Input: part model. Units: mm. Frame: model coordinates. A direction names the side the tool comes from. Give positions to 0.01 mm unless a question says otherwise; leave off trailing zeros. Loops run counter-clockwise (first coordinate to the right, second up) from the corner with the lowest first, then second, coordinate; pieces in that order, holes last. Notation, with made-up numbers: (60, 10.25) - (116, 10.25) arc R21 ccw to (116, 39.25) - close; hole circle Ø10 at (71, 58.25). An arc over 180 degrees is marked (long way). One line per item, written item: value.
from build123d import *

# Parameters (mm, degrees)
SKETCH1_R              = 6.35
SKETCH1_R_2            = 2.5527
BOSS_EXTRUDE1_DEPTH    = 9.525
FILLET1_R              = 3.175
FILLET2_R              = 1.27
F_10_32_TAPPED_HOLE1_D = 4.0386


with BuildPart() as part:
    # Sketch1 → Boss-Extrude1 (new body)
    # profile 1 of 3: a face of its own
    with BuildSketch(Plane(origin=(0, 0, 0), x_dir=(1, 0, 0), z_dir=(0, 1, 0))):
        Circle(SKETCH1_R)
        with Locations(Location((0, 0, 0), (0, 0, 90))):
            Circle(SKETCH1_R_2, mode=Mode.SUBTRACT)
    # profile 2 of 3: a face of its own
    with BuildSketch(Plane(origin=(0, 0, 0), x_dir=(1, 0, 0), z_dir=(0, 1, 0))):
        with BuildLine():
            Line((40.64, 6.35), (0, 6.35))
            ThreePointArc((0, 6.35), (4.490128061, 4.490128061), (6.35, 0))
            ThreePointArc((6.35, 0), (5.044240229, -3.857219271), (1.663971494, -6.128107283))
            Line((1.663971494, -6.128107283), (20.713971494, -0.955440505))
            ThreePointArc((20.713971494, -0.955440505), (30.971832611, -0.32456486), (40.64, -3.81))
            Line((40.64, -3.81), (40.64, 6.35))
        make_face()
    # profile 3 of 3: a face of its own
    with BuildSketch(Plane(origin=(0, 0, 0), x_dir=(1, 0, 0), z_dir=(0, 1, 0))):
        with BuildLine():
            ThreePointArc((-5.499261314, -3.175), (-6.133628997, 1.643500936), (-3.175, 5.499261314))
            Line((-3.175, 5.499261314), (-22.225, 38.494829198))
            Line((-22.225, 38.494829198), (-27.724261314, 35.319829198))
            Line((-27.724261314, 35.319829198), (-5.499261314, -3.175))
        make_face()
    extrude(amount=BOSS_EXTRUDE1_DEPTH)

    # Fillet1
    fillet1_edges = [part.edges().sort_by_distance(p)[0] for p in [
        (40.64, 4.7625, -6.35),
        (-3.175, 4.7625, -5.499261314),
        (-27.724261314, 4.7625, -35.319829198),
        (-22.225, 4.7625, -38.494829198),
    ]]
    fillet(fillet1_edges, radius=FILLET1_R - 0.0001)  # a hair under: the kernel refuses the full size

    # Fillet2
    fillet2_edges = [part.edges().sort_by_distance(p)[0] for p in [
        (40.64, 4.7625, 3.81),
    ]]
    fillet(fillet2_edges, radius=FILLET2_R)

    # #10-32 Tapped Hole1 (through all)
    with Locations(Plane(origin=(0, 9.525, 0), x_dir=(1, 0, 0), z_dir=(0, 1, 0))):
        with Locations((12.7, 1.609258642)):
            Hole(F_10_32_TAPPED_HOLE1_D / 2)


solid = part.part
Item 1: Material intervals for L1, parallel to X at y = 2.5, z = 0; L2, parallel to Z at x = 34, y = 0.75; L3, parallel to Z at x = 12.7, y = 2.75, sorted ascending.
Verdict:
L1: x = -7.33 to -2.55, 2.55 to 11.48, 13.92 to 40.64
L2: z = -6.35 to 0.95
L3: z = -6.35 to -3.63, 0.41 to 3.13
Item 2: Draft query along X for faces 3 (the face through (11.056, 4.696, 3.578)), 4 (the face through (4, 9.525, -4)), 5 (the face through (39.69, 4.83, -5.44)). Return one class per face: pulls with the +X half, pulls with the -X half, needs draft (parallel to the pull), parting line crosses it, or undercut.
Verdict:
face 3: undercut
face 4: needs draft
face 5: pulls with the +X half
Item 3: Section B-B, the plane y = 3.5. Count the separate pieces of the cut face and the enclosed holes in it, and give its area (3 significant figures).
Verdict:
separate pieces: 1
enclosed holes: 2
area: 630 mm^2
Item 4: Access query for faces 1 (the face through (19, 5, -6.35)), 2 (the face through (-0.767, 4.696, -2.435)). Directions: +Z, -Z, +X, -X, +Y, -Y. A direction counts if a zero-diameter tool reaches every point of the face in a straight line with its end or side. Return the directions, or none.
Verdict:
face 1: -Z, +X, +Y, -Y
face 2: +Y, -Y
Item 5: Section D-D, the plane x = 36. Output: boundary loops of the cut face in (y, z) (3 decimals).
Verdict:
outline: (0, -6.35) - (9.525, -6.35) - (9.525, 1.579) - (0, 1.579) - close
Item 6: Section C-C, the plane z = -7. Output: boundary loops of the cut face in (x, y) (3 decimals).
Verdict:
outline: (-11.374, 0) - (-3.859, 0) - (-3.859, 9.525) - (-11.374, 9.525) - close
Item 7: Pin query (flat end, axial travel): P1, Ø1, axis at y = 3.5, z = -27, coming from the -X side; P2, Ø3, axis at y = 8, z = -15, coming from the -X side; P3, Ø4, axis at y = 4, z = -20.5, coming from the -X side; P4, Ø1, axis at x = 26, z = -7, coming from the -Y side. Return the tip coordinate at first contact, or that it passes through.
Verdict:
P1: stops at x = -23.21
P2: stops at x = -16.86
P3: stops at x = -20.32
P4: passes through
Item 8: Section A-A, the plane x = 12.7. Output: boundary loops of the cut face in (y, z) (3 decimals), and give its area (3 significant figures).
Verdict:
outline: (0, -6.35) - (9.525, -6.35) - (9.525, -3.629) - (0, -3.629) - close; (0, 0.41) - (9.525, 0.41) - (9.525, 3.131) - (0, 3.131) - close
area: 51.8 mm^2
